from build123d import *

# Parameters (mm, degrees)
SKETCH1_R                = 2.75
BOSS_EXTRUDE1_DEPTH      = 4.7625
BOSS_EXTRUDE1_DEPTH_BACK = 4.7625
CHAMFER1_SIZE            = 3
CHAMFER2_SIZE            = 0.5


with BuildPart() as part:
    # Sketch1 → Boss-Extrude1 (new body, two sides)
    with BuildSketch(Plane.XY) as boss_extrude1_sk:
        Polygon((-170.247691321, 9.552308679), (-185.247691321, 9.552308679), (-185.247691321, 113.192388155), (-147.247691321, 113.192388155), (-147.247691321, 32.552308679), align=None)
        with Locations((-175.247691321, 66.192388155)):
            Circle(SKETCH1_R, mode=Mode.SUBTRACT)
        with Locations((-175.247691321, 86.192388155)):
            Circle(SKETCH1_R, mode=Mode.SUBTRACT)
        with Locations((-175.247691321, 106.192388155)):
            Circle(SKETCH1_R, mode=Mode.SUBTRACT)
    extrude(amount=BOSS_EXTRUDE1_DEPTH)
    extrude(boss_extrude1_sk.sketch, amount=-BOSS_EXTRUDE1_DEPTH_BACK)

    # Sketch2 → Cut-Revolve1 (revolve, cut)
    with BuildSketch(Plane.XY):
        Polygon((-165.247691321, 113.192388155), (-166.997691321, 113.192388155), (-166.997691321, 108.192388155), (-166.447691321, 107.874845507), (-166.447691321, 93.019183075), (-165.247691321, 92.326362752), align=None)
    revolve(axis=Axis((-165.247691321, 113.192388155, 0), (0, -1, 0)), mode=Mode.SUBTRACT)

    # Chamfer1
    chamfer1_edges = [part.edges().sort_by_distance(p)[0] for p in [
        (-185.247691321, 9.552308679, 0),
        (-185.247691321, 113.192388155, 0),
        (-147.247691321, 113.192388155, 0),
    ]]
    chamfer(chamfer1_edges, length=CHAMFER1_SIZE)

    # Chamfer2
    chamfer2_edges = [part.edges().sort_by_distance(p)[0] for p in [
        (-163.497691321, 113.192388155, 0),
    ]]
    chamfer(chamfer2_edges, length=CHAMFER2_SIZE)


solid = part.part
Model file for the job. Use its own axes, mm. A direction names the side the tool comes from. Coordinates: 2 decimals unless noted, no trailing zeros. Order: outer loops, then holes, each group sorted by start corner. A loop starts at its lowest first (then second) coordinate and runs counter-clockwise, first axis right, second up. Notation, with made-up numbers: (88.5, -37.5) -> (130.5, -37.5) arc R30 ccw to (130.5, -0.5) -> close; hole circle Ø8 at (-6.5, 34.25). An arc over 180 degrees is marked (long way). Return JSON: item names as keys, results as strings. Group by question number.
Item 1: Pull direction Z, two halves, no side cores. Call faces 1 (the conical face through (-165.425, 92.437, 0.073)), 2 (the flat face through (-166, 62, 4.762)), 3 (the flat face through (-185.248, 61, 0)): pulls with the +Z half, pulls with the -Z half, needs draft (parallel to the pull), parting line crosses it, or undercut.
Item 2: Tool access for faces 4 (the flat face through (-147.248, 72, 0)), 5 (the cylindrical face through (-166.917, 110.411, -0.526)): list every direction of +Z, -Z, +X, -X, +Y, -Y with a clear straight run to the whole face (end or side of a thin tool).
Item 3: Wall check: line 1 along Y through (x, z) = (-175, -2.75); line 2 along X through (y, z) = (97, 0); line 3 along X through (y, z) = (66.5, -4). Give the ranges that are in metal, low to high. Write a range as [from, to].
Item 4: Saw through at C-C on x = -159.5. Write the cut outline in (y, z).
Item 5: Flat gauge pins, fed straight in: P1, Ø1.4, axis at x = -165.25, z = 0, coming from the +Y side; P2, Ø4.5, axis at x = -165.25, z = 0, coming from the -Y side; P3, Ø5, axis at x = -175.25, y = 106.19, coming from the +Z side. Where does each tip first touch, or does it go through?
Item 6: Saw through at B-B on y = 30.5. Write the cut outline in (x, z).
Item 7: Saw through at A-A on x = -176. Write the cut outline in (y, z).
Values found:
{
 "1": {"face 1": "undercut", "face 2": "pulls with the +Z half", "face 3": "needs draft"},
 "2": {"face 4": "+Z, -Z, +X, +Y, -Y", "face 5": "+Y"},
 "3": {"line 1": "y = [9.55, 63.45], [68.93, 83.45], [88.93, 103.45], [108.93, 113.19]", "line 2": "x = [-185.25, -166.45], [-164.05, -147.25]", "line 3": "x = [-185.25, -177.98], [-172.51, -147.25]"},
 "4": {"outline": "(20.3, -4.76) -> (113.19, -4.76) -> (113.19, 4.76) -> (20.3, 4.76) -> close"},
 "5": {"P1": "stops at y = 92.73", "P2": "stops at y = 12.3", "P3": "passes through"},
 "6": {"outline": "(-185.25, -4.76) -> (-149.3, -4.76) -> (-149.3, 4.76) -> (-185.25, 4.76) -> close"},
 "7": {"outline": "(9.55, -4.76) -> (63.55, -4.76) -> (63.55, 4.76) -> (9.55, 4.76) -> close; (68.84, -4.76) -> (83.55, -4.76) -> (83.55, 4.76) -> (68.84, 4.76) -> close; (88.84, -4.76) -> (103.55, -4.76) -> (103.55, 4.76) -> (88.84, 4.76) -> close; (108.84, -4.76) -> (113.19, -4.76) -> (113.19, 4.76) -> (108.84, 4.76) -> close"}
}
